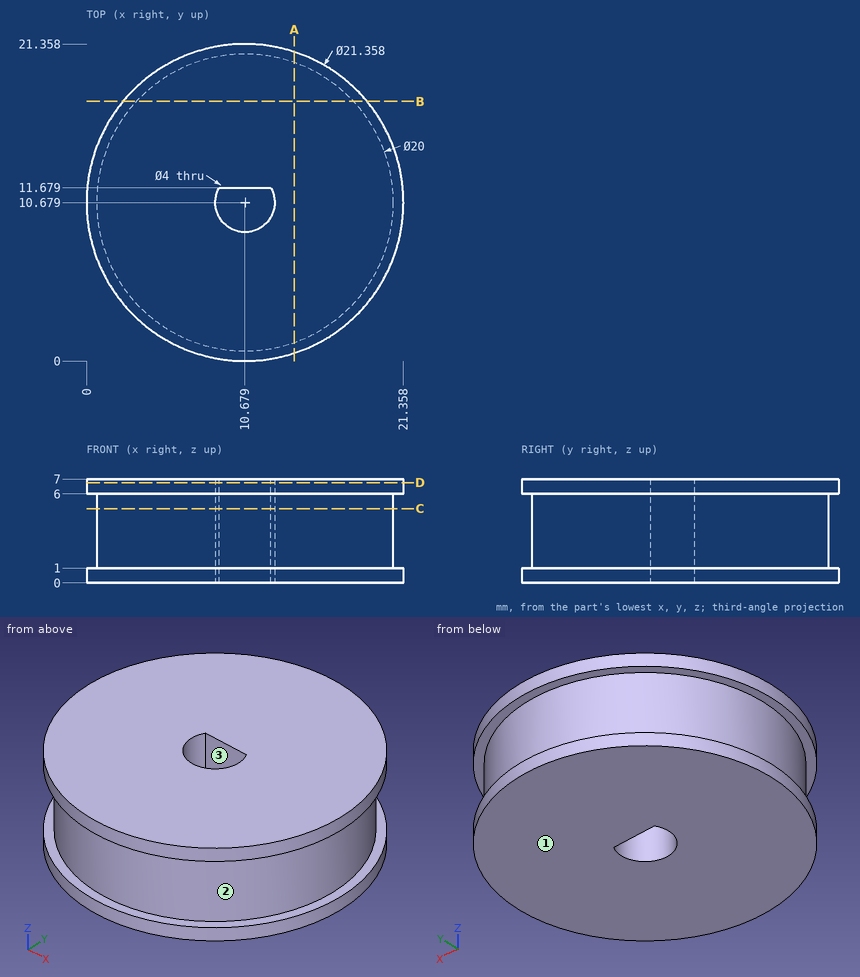
For this review, use the dimensioned drawing (mm, ordinates from the lowest corner) and the shaded views. Round coordinates to 2 decimals unless told otherwise and drop trailing zeros. Write each loop counter-clockwise with the first axis right and the second up, starting at its lowest first coordinate (ties: lowest second). Pieces come first, ordered by that corner, then holes. Notation, with made-up numbers: M -6,-18.5 L 41,-18.5 A36 cw 41,15.5 Z; hole C 47,45 d5. An arc over 180 degrees is marked long. Answer as CSV lines item,"result". Start each with the question number.
Q1. The part is to be moulded in two halves that separate along Y. For the marked faces 1, 2 and 3, say which applies: +Y half, -Y half, draft (parallel to the pull), parting line (faces both ways), or undercut.
Q2. Clearance check with flat-ended pins moving along their axes: P1, Ø2, axis at y = 7.5, z = 4.5, coming from the +X side; P2, Ø1.7, axis at x = 10.5, z = 3, coming from the -Y side; P3, Ø1, axis at x = 3.5, z = 3.5, coming from the +Y side. State where each tip first meets the part, or that it passes through.
Q3. Wall thickness on line 1 along Y through (x, z) = (10, 2.5) (1 decimal); line 2 along X through (y, z) = (9.25, 6.75) (1 decimal); line 3 along Y through (x, z) = (10.5, 3.75): over which ranges is each line inside the solid? List them lowest first.
Q4. Consider section B-B, the plane y = 17.5. Give the boundary of the cut face in (x, z), then the cut area to 3 significant figures.
Q5. Consider section C-C, the plane z = 5. Give the boundary of the cut face in (x, y), then the cut area to 3 significant figures.
Q6. Consider section A-A, the plane x = 14. Give the boundary of the cut face in (y, z), then the cut area to 3 significant figures.
Q7. Consider section D-D, the plane z = 6.75. Give the boundary of the cut face in (x, y).
Result set:
1,face 1,"draft"
1,face 2,"parting line"
1,face 3,"undercut"
2,P1,"stops at x = 20.44"
2,P2,"stops at y = 0.68"
2,P3,"stops at y = 18.12"
3,line 1,"y = 0.7 to 8.8, 11.7 to 20.7"
3,line 2,"x = 0.1 to 9.3, 12.1 to 21.3"
3,line 3,"y = 0.68 to 8.69, 11.68 to 20.68"
4,outline,"M 2.46,0 L 18.9,0 L 18.9,1 L 17.99,1 L 17.99,6 L 18.9,6 L 18.9,7 L 2.46,7 L 2.46,6 L 3.37,6 L 3.37,1 L 2.46,1 Z"
4,area,"106 mm²"
5,outline,"C 10.68,10.68 d20; hole M 8.95,11.68 A2 ccw long 12.41,11.68 Z"
5,area,"304 mm²"
6,outline,"M 0.53,0 L 20.83,0 L 20.83,1 L 20.11,1 L 20.11,6 L 20.83,6 L 20.83,7 L 0.53,7 L 0.53,6 L 1.25,6 L 1.25,1 L 0.53,1 Z"
6,area,"135 mm²"
7,outline,"C 10.68,10.68 d21.36; hole M 8.95,11.68 A2 ccw long 12.41,11.68 Z"
